```python
from build123d import *

# Parameters (mm, degrees)
SKETCH1_R                      = 8.73125
BOSS_EXTRUDE1_DEPTH            = 6.35
SKETCH7_R                      = 7.235
SKETCH7_R_2                    = 4.435
CUT_EXTRUDE2_DEPTH             = 2.000000064
M3_CLEARANCE_HOLE2_D           = 3.4
F_2_0_221_DIAMETER_HOLE1_D     = 5.6134
F_2_0_221_DIAMETER_HOLE1_DEPTH = 6.35
F_1_4_CLEARANCE_HOLE2_D        = 6.7564
TAP_DRILL_FOR_2_56_TAP2_D      = 1.778
TAP_DRILL_FOR_2_56_TAP2_DEPTH  = 12.7
TAP_DRILL_FOR_2_56_TAP2_TIP    = 0.53416509
FILLET1_R                      = 6.35
TAP_DRILL_FOR_2_56_TAP1_D      = 1.778


with BuildPart() as part:
    # Sketch1 → Boss-Extrude1 (new body)
    with BuildSketch(Plane(origin=(0, 0, 0), x_dir=(0, 0, -1), z_dir=(1, 0, 0))):
        with BuildLine():
            Line((34.282198326, -22.486920134), (34.282198326, 133.723079866))
            Line((34.282198326, 133.723079866), (-41.917801674, 133.723079866))
            Line((-41.917801674, 133.723079866), (-41.917801674, -22.486920134))
            ThreePointArc((-41.917801674, -22.486920134), (-40.057929734, -26.977048194), (-35.567801674, -28.836920134))
            Line((-35.567801674, -28.836920134), (27.932198326, -28.836920134))
            ThreePointArc((27.932198326, -28.836920134), (32.422326387, -26.977048194), (34.282198326, -22.486920134))
        make_face()
        with Locations((-3.817801674, 21.963079866)):
            Circle(SKETCH1_R, mode=Mode.SUBTRACT)
    extrude(amount=BOSS_EXTRUDE1_DEPTH)

    # Sketch7 → Cut-Extrude2 (cut)
    with BuildSketch(Plane(origin=(6.35, 0, 0), x_dir=(0, 0, -1), z_dir=(1, 0, 0))):
        with Locations((-3.817801674, 21.963079866)):
            Circle(SKETCH7_R)
        with Locations((3.388972242, 32.920368331)):
            Circle(SKETCH7_R_2)
        with Locations((-14.337567313, 29.794701133)):
            Circle(SKETCH7_R_2)
        with Locations((9.119362105, 0.421712482)):
            Circle(SKETCH7_R_2)
        with Locations((-8.60717745, -2.703954716)):
            Circle(SKETCH7_R_2)
        with BuildLine():
            Line((-7.135844138, 12.274719881), (2.613752617, 13.99383684))
            ThreePointArc((2.613752617, 13.99383684), (6.824739925, 11.045271784), (3.876174868, 6.834284476))
            Line((3.876174868, 6.834284476), (-5.873421887, 5.115167517))
            ThreePointArc((-5.873421887, 5.115167517), (-10.084409195, 8.063732573), (-7.135844138, 12.274719881))
        make_face()
    extrude(amount=-CUT_EXTRUDE2_DEPTH, mode=Mode.SUBTRACT)

    # M3 Clearance Hole2 (through all)
    with Locations(Plane(origin=(6.35, 0, 0), x_dir=(0, 0, -1), z_dir=(1, 0, 0))):
        with Locations((9.119362105, 0.421712482), (-8.60717745, -2.703954716), (-14.337567313, 29.794701133), (3.388972242, 32.920368331)):
            Hole(M3_CLEARANCE_HOLE2_D / 2)

    # #2 (0.221) Diameter Hole1
    with Locations(Plane.ZY):
        with Locations((-22.828731326, 123.563340866), (31.159813674, 123.563340866), (31.159813674, 52.443340866), (-22.828731326, 52.443340866), (-22.828731326, -18.676659134), (31.159813674, -18.676659134)):
            Hole(F_2_0_221_DIAMETER_HOLE1_D / 2, depth=F_2_0_221_DIAMETER_HOLE1_DEPTH)

    # 1/4 Clearance Hole2 (through all)
    with Locations(Plane(origin=(6.35, 0, 0), x_dir=(0, 0, -1), z_dir=(1, 0, 0))):
        with Locations((-3.817801674, 72.763079866)):
            Hole(F_1_4_CLEARANCE_HOLE2_D / 2)

    # Tap Drill for #2-56 Tap2
    with Locations(Plane(origin=(0, 167.140830498, -34.282198326), x_dir=(1, 0, 0), z_dir=(0, 0, -1))):
        with Locations((3.175, 58.817489631), (3.175, 79.137489631)):
            Hole(TAP_DRILL_FOR_2_56_TAP2_D / 2, depth=TAP_DRILL_FOR_2_56_TAP2_DEPTH)
            with Locations((0, 0, -(TAP_DRILL_FOR_2_56_TAP2_DEPTH + TAP_DRILL_FOR_2_56_TAP2_TIP / 2))):  # 118° drill point
                Cone(0, TAP_DRILL_FOR_2_56_TAP2_D / 2, TAP_DRILL_FOR_2_56_TAP2_TIP, mode=Mode.SUBTRACT)

    # Fillet1
    fillet1_edges = [part.edges().sort_by_distance(p)[0] for p in [
        (3.175, 133.723079866, 41.917801674),
        (3.175, 133.723079866, -34.282198326),
    ]]
    fillet(fillet1_edges, radius=FILLET1_R)

    # Tap Drill for #2-56 Tap1 (through all)
    with Locations(Plane(origin=(6.35, 0, 0), x_dir=(0, 0, -1), z_dir=(1, 0, 0))):
        with Locations((6.432198326, 130.157875406), (-32.567801674, 130.157875406)):
            Hole(TAP_DRILL_FOR_2_56_TAP1_D / 2)


solid = part.part
```
Part model, mm, in its own coordinate system. A direction names the side the tool comes from. Coordinates: 2 decimals unless noted, no trailing zeros. Write each loop counter-clockwise with the first axis right and the second up, starting at its lowest first coordinate (ties: lowest second). Pieces come first, ordered by that corner, then holes.
Item 1: Slice it at B-B (x = 1). Count the separate pieces of the cut face and the enclosed holes in it, and give its area (3 significant figures).
Item 2: Mould opens along Z. For faces 1 (the face through (3.131, -26.927, 40.107)), 2 (the face through (3.219, 131.814, -32.471)), 3 (the face through (3.219, -21.417, -22.22)) say: released by +Z, released by -Z, zero draft, split by the parting line, or undercut.
Item 3: Pin check, flat tips, straight feed: pin 1 (3 mm diameter, centred on y = -2.7, z = 8.61, fed in from +X); pin 2 (5.5 mm diameter, centred on y = 0.42, z = -9.12, fed in from +X). Stop position of each tip, or through.
Item 4: Probe line 1 (Z direction, x = 2.75, y = 29.5); line 2 (Y direction, x = 5, z = 5); line 3 (Y direction, x = 6, z = -12). List the from-to ranges inside material, lowest first.
Item 5: Which spindle directions (+Z, -Z, +X, -X, +Y, -Y) get a long thin tool onto all of the face, cutting with end or side? Do faces 4 (the face through (2.14, 34.07, -4.64)), 5 (the face through (5.36, -4.4, 4.51)). Say none if no direction does.
Item 6: Slice it at A-A (z = -23.5). Write the cut outline in (x, y) (3 decimals), and give its area (3 significant figures).
Results found:
1. separate pieces: 1
1. enclosed holes: 14
1. area: 11,900 mm2
2. face 1: released by +Z
2. face 2: released by -Z
2. face 3: undercut
3. pin 1: passes through
3. pin 2: stops at x = 4.35
4. line 1: z = -34.28 to -0.59, 8.23 to 12.66, 16.01 to 41.92
4. line 2: y = -28.84 to -5.28, -0.12 to 5.27, 12.65 to 13.31, 30.61 to 69.6, 75.93 to 133.72
4. line 3: y = -28.84 to -2.95, 3.79 to 133.72
5. face 4: +X, -X
5. face 5: +X
6. outline: (0, -28.837) - (6.35, -28.837) - (6.35, -21.402) - (0, -21.402) - close; (0, -15.951) - (6.35, -15.951) - (6.35, 49.718) - (0, 49.718) - close; (0, 55.169) - (6.35, 55.169) - (6.35, 120.838) - (0, 120.838) - close; (0, 126.289) - (6.35, 126.289) - (6.35, 133.723) - (0, 133.723) - close; hole circle Ø1.778 at (3.175, 88.003); hole circle Ø1.778 at (3.175, 108.323)
6. area: 923 mm2
